Autodesk Inventor part; units mm, degrees
ref_plane "YZ Plane" through (0, 0, 0) normal (1, 0, 0) x (0, 1, 0)
ref_plane "XZ Plane" through (0, 0, 0) normal (0, 1, 0) x (-1, 0, 0)
ref_plane "XY Plane" through (0, 0, 0) normal (0, 0, 1) x (1, 0, 0)
sketch "Sketch1" plane through (0, 0, 0) normal (0, 0, 1) x (1, 0, 0)
  line L0 (31.3464, 73.7708) -> (86.3464, 73.7708)
  line L1 (86.3464, 73.7708) -> (86.3464, 38.7708)
  line L2 (86.3464, 38.7708) -> (31.3464, 38.7708)
  line L3 (31.3464, 38.7708) -> (31.3464, 73.7708)
  circle A0 centre (43.3464, 56.2708) radius 2.5
  point P0 (0, 0)
  dimension "d0" = 55
  dimension "d1" = 35
  dimension "d3" = 5
extrude "Extrusion1" add sketch "Sketch1" along normal blind 2
sketch "Sketch2" plane through (0, 0, 2) normal (0, 0, 1) x (1, 0, 0)
  point P0 (0, 0)
thread "Thread1"
sketch "Sketch3" plane through (86.3464, 38.7708, 0) normal (1, 0, 0) x (0, 0, -1)
  point P0 (0, -38.7708)
sketch "Sketch4" plane through (0, 0, 2) normal (0, 0, 1) x (1, 0, 0)
  point P0 (0, 0)
sketch "Sketch5" plane through (86.3464, 38.7708, 0) normal (1, 0, 0) x (0, 0, -1)
  line L0 (-2, 0) -> (-2, 35)
  line L1 (-2, 35) -> (0, 35)
  line L2 (0, 35) -> (0, 0)
  line L3 (0, 0) -> (-2, 0)
  line L4 (-2, 0) -> (-2, 35)
  point P0 (0, -38.7708)
  dimension "d8" = 2
  dimension "d9" = 35
extrude "Extrusion2" cut sketch "Sketch5" against normal blind 15
sketch "Sketch6" plane through (0, 0, 2) normal (0, 0, 1) x (1, 0, 0)
  line L0 (31.3464, 38.7708) -> (71.3464, 38.7708)
  line L1 (31.3464, 38.7708) -> (71.3464, 38.7708)
  line L2 (71.3464, 38.7708) -> (71.3464, 43.7708)
  line L3 (71.3464, 43.7708) -> (31.3464, 43.7708)
  line L4 (31.3464, 43.7708) -> (31.3464, 38.7708)
  point P0 (0, 0)
  dimension "d12" = 40
  dimension "d13" = 5
extrude "Extrusion3" cut sketch "Sketch6" against normal blind 15
sketch "Sketch7" plane through (0, 0, 0) normal (0, 0, -1) x (-1, 0, 0)
  line L0 (-71.3464, 73.7708) -> (-31.3464, 73.7708)
  line L1 (-71.3464, 73.7708) -> (-31.3464, 73.7708)
  line L2 (-31.3464, 73.7708) -> (-31.3464, 68.7708)
  line L3 (-31.3464, 68.7708) -> (-71.3464, 68.7708)
  line L4 (-71.3464, 68.7708) -> (-71.3464, 73.7708)
  point P0 (0, 0)
  dimension "d16" = 40
  dimension "d17" = 5
extrude "Extrusion4" cut sketch "Sketch7" against normal blind 15
properties part number "Peyangga Samping Kamera"
Geometry check sheet. Reference: the model listing, model coordinates, mm. Round coordinates to 2 decimals unless told otherwise and drop trailing zeros. Order: outer loops, then holes, each group sorted by start corner. A loop starts at its lowest first (then second) coordinate and runs counter-clockwise, first axis right, second up. Notation, with made-up numbers: M -32.75,46.5 L -23.75,46.5 A28 cw -23.75,84.5 Z; hole C -25.75,-2 d7. An arc over 180 degrees is marked long. Answer in a Markdown table with one row per item. Add a question column.
Item 1: Sectioned sample at B-B, the plane z = 1.4. Enter the section's corners in (x, y).
Item 2: Depth check by flat-ended pin: pin 1 Ø6 at (x, y) = (43.5, 54.5) entering from +Z; pin 2 Ø3 at (x, y) = (43.35, 56.27) entering from -Z. Enter the tip coordinate at first touch or a pass-through.
Item 3: Sectioned sample at A-A, the plane x = 42.5. Enter the section's corners in (y, z).
Item 4: Draft check along X on faces 1 (the face through (41.504, 54.581, 0.986)), 2 (the face through (71.346, 56, 1)), 3 (the face through (31.346, 56, 1)), 4 (the face through (51, 56, 2)). Enter one of: released by +X, released by -X, zero draft, split by the parting line, or undercut.
Item 5: Material ranges on L1, parallel to X at y = 55.5, z = 0.1; L2, parallel to X at y = 57.5, z = 0.7, recorded low to high. Write a range as [from, to].
Filled in:
| question | item | result |
|---|---|---|
| 1 | outline | M 31.35,43.77 L 71.35,43.77 L 71.35,68.77 L 31.35,68.77 Z; hole C 43.35,56.27 d5 |
| 2 | pin 1 | stops at z = 2 |
| 2 | pin 2 | passes through |
| 3 | outline | M 43.77,0 L 53.92,0 L 53.92,2 L 43.77,2 Z; M 58.62,0 L 68.77,0 L 68.77,2 L 58.62,2 Z |
| 4 | face 1 | undercut |
| 4 | face 2 | released by +X |
| 4 | face 3 | released by -X |
| 4 | face 4 | zero draft |
| 5 | L1 | x = [31.35, 40.97], [45.72, 71.35] |
| 5 | L2 | x = [31.35, 41.17], [45.52, 71.35] |
